Design review of the part built by this model. Coordinates are the model's own, in mm. Face numbers are marked on the shaded views. A direction names the side the tool comes from. Give positions to 0.01 mm unless a question says otherwise; leave off trailing zeros. Write each loop counter-clockwise with the first axis right and the second up, starting at its lowest first coordinate (ties: lowest second). Pieces come first, ordered by that corner, then holes. Notation, with made-up numbers: (-15, -32) -> (35, -32) arc R35 cw to (35, 5) -> close; hole circle Ø4 at (66.5, 0). An arc over 180 degrees is marked (long way). Answer as a JSON object with one key per item and string values.
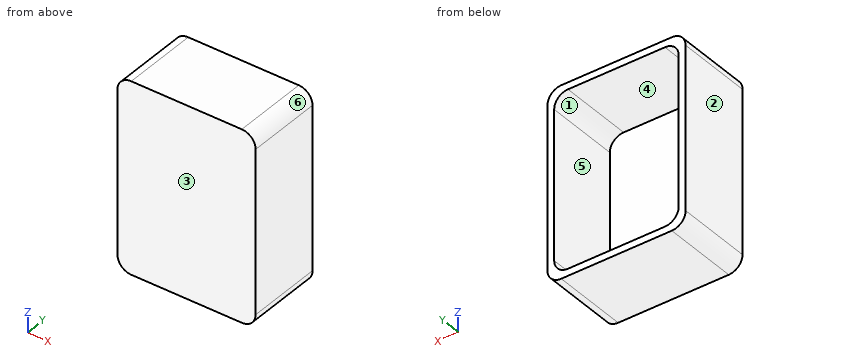
```python
from build123d import *

# Parameters (mm, degrees)
SKETCH1_W           = 400
SKETCH1_H           = 550
BOSS_EXTRUDE1_DEPTH = 220
SKETCH2_W           = 360.460384802
SKETCH2_H           = 509.949814821
CUT_EXTRUDE1_DEPTH  = 215
FILLET2_R           = 40
FILLET3_R           = 40


with BuildPart() as part:
    # Sketch1 → Boss-Extrude1 (new body)
    with BuildSketch(Plane(origin=(0, 0, 0), x_dir=(1, 0, 0), z_dir=(0, 1, 0))):
        Rectangle(SKETCH1_W, SKETCH1_H)
    extrude(amount=BOSS_EXTRUDE1_DEPTH)

    # Sketch2 → Cut-Extrude1 (cut)
    with BuildSketch(Plane(origin=(0, 220, 0), x_dir=(1, 0, 0), z_dir=(0, 1, 0))):
        with Locations((0.230192401, -0.02509259)):
            Rectangle(SKETCH2_W, SKETCH2_H)
    extrude(amount=-CUT_EXTRUDE1_DEPTH, mode=Mode.SUBTRACT)

    # Fillet2
    fillet2_edges = [part.edges().sort_by_distance(p)[0] for p in [
        (200, 110, 275),
        (-200, 110, 275),
        (-200, 110, -275),
        (200, 110, -275),
    ]]
    fillet(fillet2_edges, radius=FILLET2_R)

    # Fillet3
    fillet3_edges = [part.edges().sort_by_distance(p)[0] for p in [
        (180.460384802, 112.5, -254.949814821),
        (180.460384802, 112.5, 255),
        (-180, 112.5, 255),
        (-180, 112.5, -254.949814821),
    ]]
    fillet(fillet3_edges, radius=FILLET3_R)


solid = part.part
```
(1) For the marked faces 1 and 2, list the 3-axis set-ups (+Z, -Z, +X, -X, +Y, -Y) from which the entire face can be reached by the end or side of a thin tool; tool diameter is ignored.
Here are the results:
{"face 1": "+Y", "face 2": "+Z, -Z, -X, +Y, -Y"}
(2) We need section B-B, the plane y = 137. State the section outline as (x, z) points.
Here are the results:
{"outline": "(-200, -235) arc R40 ccw to (-160, -275) -> (160, -275) arc R40 ccw to (200, -235) -> (200, 235) arc R40 ccw to (160, 275) -> (-160, 275) arc R40 ccw to (-200, 235) -> close; hole (-180, -214.95) arc R40 ccw to (-140, -254.95) -> (140.46, -254.95) arc R40 ccw to (180.46, -214.95) -> (180.46, 215) arc R40 ccw to (140.46, 255) -> (-140, 255) arc R40 ccw to (-180, 215) -> close"}
(3) For line 1 along X through (y, z) = (133, 58.5); line 2 along Z through (x, y) = (100, 90); line 3 along X through (y, z) = (89.5, 218), list the stretches that pass through material, from the lowest coordinate up.
Here are the results:
{"line 1": "x = -200 to -180, 180.46 to 200", "line 2": "z = -275 to -254.95, 255 to 275", "line 3": "x = -200 to -179.89, 180.35 to 200"}
(4) The part is to be moulded in two halves that separate along Z. For the marked faces 3, 4, 5 and 6, say which applies: +Z half, -Z half, draft (parallel to the pull), parting line (faces both ways), or undercut.
Here are the results:
{"face 3": "draft", "face 4": "undercut", "face 5": "undercut", "face 6": "+Z half"}
(5) We need section A-A, the plane z = 126. State the section outline as (x, y) points.
Here are the results:
{"outline": "(-200, 0) -> (200, 0) -> (200, 220) -> (180.46, 220) -> (180.46, 5) -> (-180, 5) -> (-180, 220) -> (-200, 220) -> close"}
(6) Clearance check with a flat-ended pin moving along its axis: pin 1 (2 mm diameter, centred on x = -73.5, z = -85, fed in from +Y). State where the tip first meets the part, or that it passes through.
Here are the results:
{"pin 1": "stops at y = 5"}
(7) We need section C-C, the plane x = 10.5. State the section outline as (y, z) points, then the cut area to 3 significant figures.
Here are the results:
{"outline": "(0, -275) -> (220, -275) -> (220, -254.95) -> (5, -254.95) -> (5, 255) -> (220, 255) -> (220, 275) -> (0, 275) -> close", "area": "11,400 mm²"}
